For this review, take the finished solid that the model builds, in its own axes (mm). Face numbers are marked on the shaded views. A direction names the side the tool comes from. Give positions to 0.01 mm unless a question says otherwise; leave off trailing zeros. Order: outer loops, then holes, each group sorted by start corner. A loop starts at its lowest first (then second) coordinate and runs counter-clockwise, first axis right, second up. Notation, with made-up numbers: (36.25, 35) -> (93.25, 35) arc R20 ccw to (93.25, 70) -> close; hole circle Ø1 at (-32, -18). An arc over 180 degrees is marked (long way). Return JSON: item names as keys, results as strings. Group by question number.
1) Add section C-C (y = 26). Give the boundary of the cut face in (x, z).
2) Insertion check: P1, Ø1.5, axis at x = 7.5, z = 20.5, coming from the -Y side; P2, Ø10, axis at x = -25, y = 12, coming from the +Z side; P3, Ø12, axis at x = -1.5, z = 13, coming from the -Y side. Each pin has a flat end and moves straight along its axis. Give the tip position at first contact, or say it passes through.
3) The part is to be moulded in two halves that separate along Y. For the marked faces 4, 5 and 6, say which applies: released by +Y, released by -Y, zero draft, split by the parting line, or undercut.
4) Add section D-D (z = -24). Give the boundary of the cut face in (x, y), then the cut area to 3 significant figures.
5) For the marked faces 1, 2 and 3, list the 3-axis set-ups (+Z, -Z, +X, -X, +Y, -Y) from which the entire face can be reached by the end or side of a thin tool; tool diameter is ignored.
6) To check wall thickness, follow line 1 along Y through (x, z) = (0, 1); line 2 along Y through (x, z) = (26, -14.5); line 3 along X through (y, z) = (22, -20). State the ranges of each line that lie inside material, in increasing order.
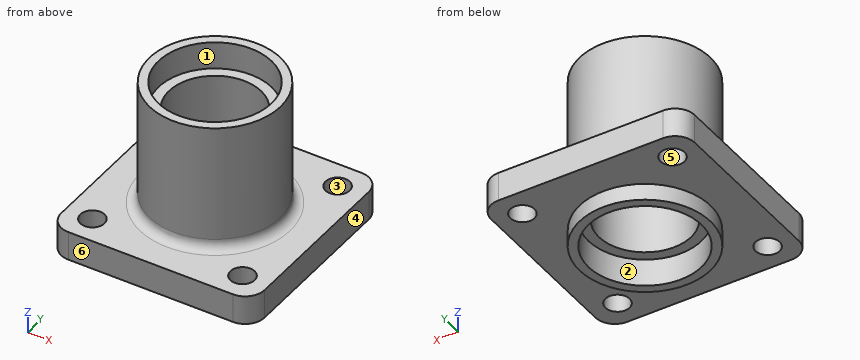
from build123d import *

# Parameters (mm, degrees)
SKETCH1_R                = 21.43125
SKETCH1_R_2              = 15.08125
BOSS_EXTRUDE1_DEPTH      = 28.2575
BOSS_EXTRUDE1_DEPTH_BACK = 28.2575
SKETCH2_R                = 3.96875
SKETCH2_R_2              = 20.6375
BOSS_EXTRUDE2_DEPTH      = 9.525
SKETCH3_R                = 18.5
CUT_EXTRUDE1_DEPTH       = 9
FILLET1_R                = 3.175


with BuildPart() as part:
    # Sketch1 → Boss-Extrude1 (new body, two sides)
    with BuildSketch(Plane.XY) as boss_extrude1_sk:
        Circle(SKETCH1_R)
        Circle(SKETCH1_R_2, mode=Mode.SUBTRACT)
    extrude(amount=BOSS_EXTRUDE1_DEPTH)
    extrude(boss_extrude1_sk.sketch, amount=-BOSS_EXTRUDE1_DEPTH_BACK)

    # Sketch2 → Boss-Extrude2 (add)
    with BuildSketch(Plane.XY.offset(-22.7965)):
        with BuildLine():
            Line((-26.9875, 33.3375), (26.9875, 33.3375))
            ThreePointArc((26.9875, 33.3375), (31.477628061, 31.477628061), (33.3375, 26.9875))
            Line((33.3375, 26.9875), (33.3375, -26.9875))
            ThreePointArc((33.3375, -26.9875), (31.477628061, -31.477628061), (26.9875, -33.3375))
            Line((26.9875, -33.3375), (-26.9875, -33.3375))
            ThreePointArc((-26.9875, -33.3375), (-31.477628061, -31.477628061), (-33.3375, -26.9875))
            Line((-33.3375, -26.9875), (-33.3375, 26.9875))
            ThreePointArc((-33.3375, 26.9875), (-31.477628061, 31.477628061), (-26.9875, 33.3375))
        make_face()
        with Locations((-24.60625, 24.60625)):
            Circle(SKETCH2_R, mode=Mode.SUBTRACT)
        with Locations((24.60625, 24.60625)):
            Circle(SKETCH2_R, mode=Mode.SUBTRACT)
        with Locations((24.60625, -24.60625)):
            Circle(SKETCH2_R, mode=Mode.SUBTRACT)
        with Locations((-24.60625, -24.60625)):
            Circle(SKETCH2_R, mode=Mode.SUBTRACT)
        Circle(SKETCH2_R_2, mode=Mode.SUBTRACT)
    extrude(amount=BOSS_EXTRUDE2_DEPTH)

    # Sketch3 → Cut-Extrude1 (cut)
    with BuildSketch(Plane.XY.offset(28.2575)):
        Circle(SKETCH3_R)
    cut_extrude1 = extrude(amount=-CUT_EXTRUDE1_DEPTH, mode=Mode.SUBTRACT)

    # Mirror1: Cut-Extrude1 across plane
    add(cut_extrude1.mirror(Plane.XY), mode=Mode.SUBTRACT)

    # Fillet1
    fillet1_edges = [part.edges().sort_by_distance(p)[0] for p in [
        (-21.43125, 0, -13.2715),
    ]]
    fillet(fillet1_edges, radius=FILLET1_R)


solid = part.part
Evaluation:
{
 "1": {"outline": "(-33.34, -22.8) -> (-28.32, -22.8) -> (-28.32, -13.27) -> (-33.34, -13.27) -> close; (-20.89, -22.8) -> (20.89, -22.8) -> (20.89, -13.27) -> (-20.89, -13.27) -> close; (28.32, -22.8) -> (33.34, -22.8) -> (33.34, -13.27) -> (28.32, -13.27) -> close"},
 "2": {"P1": "y = -20.34", "P2": "z = -12.66", "P3": "y = -21.43"},
 "3": {"face 4": "zero draft", "face 5": "undercut", "face 6": "released by -Y"},
 "4": {"outline": "circle Ø42.86 at (0, 0); hole circle Ø37 at (0, 0)", "area": "368 mm^2"},
 "5": {"face 1": "+Z", "face 2": "-Z", "face 3": "+Z, -Z"},
 "6": {"line 1": "-21.43 to -15.08, 15.08 to 21.43", "line 2": "-33.34 to -28.32, -20.89 to 20.89, 28.32 to 33.34", "line 3": "-33.34 to -27.6, -21.61 to 21.61, 27.6 to 33.34"}
}
